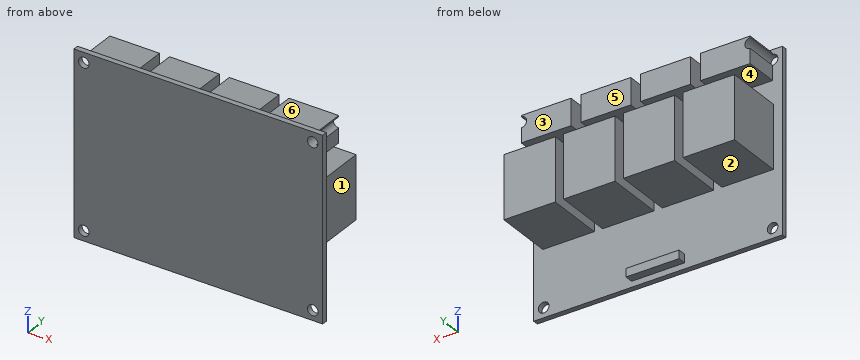
from build123d import *

# Parameters (mm, degrees)
SKETCH1_W              = 75
SKETCH1_H              = 55
PCB_DEPTH              = 1.6
RELAY_1_START          = 1.6
SKETCH2_W              = 15.5
SKETCH2_H              = 19
RELAY_1_DEPTH          = 17.4
TERMINAL_1_START       = 1.6
SKETCH3_W              = 15
SKETCH3_H              = 8
TERMINAL_1_DEPTH       = 10
RELAY_2_START          = 1.6
SKETCH4_W              = 15.5
SKETCH4_H              = 19
RELAY_2_DEPTH          = 17.4
TERMINAL_2_START       = 1.6
SKETCH5_W              = 15
SKETCH5_H              = 8
TERMINAL_2_DEPTH       = 10
RELAY_3_START          = 1.6
SKETCH6_W              = 15.5
SKETCH6_H              = 19
RELAY_3_DEPTH          = 17.4
TERMINAL_3_START       = 1.6
SKETCH7_W              = 15
SKETCH7_H              = 8
TERMINAL_3_DEPTH       = 10
RELAY_4_START          = 1.6
SKETCH8_W              = 15.5
SKETCH8_H              = 19
RELAY_4_DEPTH          = 17.4
TERMINAL_4_START       = 1.6
SKETCH9_W              = 15
SKETCH9_H              = 8
TERMINAL_4_DEPTH       = 10
HEADER_START           = 1.6
SKETCH10_W             = 16
SKETCH10_H             = 2.5
HEADER_DEPTH           = 2.5
MOUNT_HOLES_DEPTH      = 51.23445033
MOUNT_HOLES_DEPTH_BACK = 51.23445033
SKETCH11_R             = 1.6


with BuildPart() as part:
    # Sketch1 → PCB (new body)
    with BuildSketch(Plane(origin=(0, 0, 0), x_dir=(1, 0, 0), z_dir=(0, 1, 0))):
        Rectangle(SKETCH1_W, SKETCH1_H)
    extrude(amount=PCB_DEPTH)

    # Sketch2 → Relay_1 (add)
    with BuildSketch(Plane(origin=(0, 0, 0), x_dir=(1, 0, 0), z_dir=(0, 1, 0)).offset(RELAY_1_START)):
        with Locations((-27, -2)):
            Rectangle(SKETCH2_W, SKETCH2_H)
    extrude(amount=RELAY_1_DEPTH)

    # Sketch3 → Terminal_1 (add)
    with BuildSketch(Plane(origin=(0, 0, 0), x_dir=(1, 0, 0), z_dir=(0, 1, 0)).offset(TERMINAL_1_START)):
        with Locations((-27, -22.5)):
            Rectangle(SKETCH3_W, SKETCH3_H)
    extrude(amount=TERMINAL_1_DEPTH)

    # Sketch4 → Relay_2 (add)
    with BuildSketch(Plane(origin=(0, 0, 0), x_dir=(1, 0, 0), z_dir=(0, 1, 0)).offset(RELAY_2_START)):
        with Locations((-9, -2)):
            Rectangle(SKETCH4_W, SKETCH4_H)
    extrude(amount=RELAY_2_DEPTH)

    # Sketch5 → Terminal_2 (add)
    with BuildSketch(Plane(origin=(0, 0, 0), x_dir=(1, 0, 0), z_dir=(0, 1, 0)).offset(TERMINAL_2_START)):
        with Locations((-9, -22.5)):
            Rectangle(SKETCH5_W, SKETCH5_H)
    extrude(amount=TERMINAL_2_DEPTH)

    # Sketch6 → Relay_3 (add)
    with BuildSketch(Plane(origin=(0, 0, 0), x_dir=(1, 0, 0), z_dir=(0, 1, 0)).offset(RELAY_3_START)):
        with Locations((9, -2)):
            Rectangle(SKETCH6_W, SKETCH6_H)
    extrude(amount=RELAY_3_DEPTH)

    # Sketch7 → Terminal_3 (add)
    with BuildSketch(Plane(origin=(0, 0, 0), x_dir=(1, 0, 0), z_dir=(0, 1, 0)).offset(TERMINAL_3_START)):
        with Locations((9, -22.5)):
            Rectangle(SKETCH7_W, SKETCH7_H)
    extrude(amount=TERMINAL_3_DEPTH)

    # Sketch8 → Relay_4 (add)
    with BuildSketch(Plane(origin=(0, 0, 0), x_dir=(1, 0, 0), z_dir=(0, 1, 0)).offset(RELAY_4_START)):
        with Locations((27, -2)):
            Rectangle(SKETCH8_W, SKETCH8_H)
    extrude(amount=RELAY_4_DEPTH)

    # Sketch9 → Terminal_4 (add)
    with BuildSketch(Plane(origin=(0, 0, 0), x_dir=(1, 0, 0), z_dir=(0, 1, 0)).offset(TERMINAL_4_START)):
        with Locations((27, -22.5)):
            Rectangle(SKETCH9_W, SKETCH9_H)
    extrude(amount=TERMINAL_4_DEPTH)

    # Sketch10 → Header (add)
    with BuildSketch(Plane(origin=(0, 0, 0), x_dir=(1, 0, 0), z_dir=(0, 1, 0)).offset(HEADER_START)):
        with Locations((0, 24.5)):
            Rectangle(SKETCH10_W, SKETCH10_H)
    extrude(amount=HEADER_DEPTH)

    # Sketch11 → Mount_Holes (cut, two sides: drawn at the far end of the back side and taken through both)
    with BuildSketch(Plane(origin=(0, 0, 0), x_dir=(1, 0, 0), z_dir=(0, 1, 0)).offset(-MOUNT_HOLES_DEPTH_BACK)):
        with Locations(Location((-34.5, 24.5, 0), (0, 0, 90))):
            Circle(SKETCH11_R)
        with Locations(Location((-34.5, -24.5, 0), (0, 0, 270))):
            Circle(SKETCH11_R)
        with Locations(Location((34.5, 24.5, 0), (0, 0, 90))):
            Circle(SKETCH11_R)
        with Locations(Location((34.5, -24.5, 0), (0, 0, 270))):
            Circle(SKETCH11_R)
    extrude(amount=MOUNT_HOLES_DEPTH + MOUNT_HOLES_DEPTH_BACK, mode=Mode.SUBTRACT)


solid = part.part
Geometry: final body of the model. Coordinates: model frame, mm. Face numbers are marked on the shaded views. A direction names the side the tool comes from. Coordinates: 2 decimals unless noted, no trailing zeros. Order: outer loops, then holes, each group sorted by start corner. A loop starts at its lowest first (then second) coordinate and runs counter-clockwise, first axis right, second up.
(1) Access query for the marked faces 1, 2 and 3. Directions: +Z, -Z, +X, -X, +Y, -Y. A direction counts if a zero-diameter tool reaches every point of the face in a straight line with its end or side. Return the directions, or none.
(2) Material intervals for probe 1 along X at (y, z) = (3.5, 24.5); probe 2 along X at (y, z) = (2.5, 0.5); probe 3 along X at (y, z) = (1.25, -24.5), sorted ascending.
(3) Draft query along Z for the marked faces 4, 5 and 6. Return one class per face: pulls with the +Z half, pulls with the -Z half, needs draft (parallel to the pull), parting line crosses it, or undercut.
(4) First-contact query: pin 1 (1 mm diameter, centred on x = 0.5, y = 11.5, fed in from -Z); pin 2 (5 mm diameter, centred on x = -12.5, y = 8, fed in from -Z); pin 3 (2.5 mm diameter, centred on y = 5.5, z = 23.5, fed in from -X); pin 4 (1.5 mm diameter, centred on x = 8.5, z = -18.5, fed in from +Y). Flat tips, straight axial feed; report the tip coordinate or a pass-through.
(5) Section query C-C (x = 21). Return the cut outline in (y, z), plus the area to 3 significant figures.
(6) Section query B-B (z = 24.5). Return the cut outline in (x, y).
(7) Section query A-A (y = 13.5). Return the cut outline in (x, z), plus the area to 3 significant figures.
(8) Section query D-D (z = -5). Return the cut outline in (x, y), plus the area to 3 significant figures.
Solution:
1. face 1: +Z, -Z, +X, +Y
1. face 2: -Z, +X, -X, +Y
1. face 3: +Z, +X, -X, +Y
2. probe 1: x = -32.9 to -19.5, -16.5 to -1.5, 1.5 to 16.5, 19.5 to 32.9
2. probe 2: x = -34.75 to -19.25, -16.75 to -1.25, 1.25 to 16.75, 19.25 to 34.75
2. probe 3: x = -37.5 to -36.1, -32.9 to 32.9, 36.1 to 37.5
3. face 4: undercut
3. face 5: needs draft
3. face 6: pulls with the +Z half
4. pin 1: passes through
4. pin 2: stops at z = -7.5
4. pin 3: stops at x = -34.5
4. pin 4: stops at y = 1.6
5. outline: (0, -27.5) - (1.6, -27.5) - (1.6, -7.5) - (19, -7.5) - (19, 11.5) - (1.6, 11.5) - (1.6, 18.5) - (11.6, 18.5) - (11.6, 26.5) - (1.6, 26.5) - (1.6, 27.5) - (0, 27.5) - close
5. area: 499 mm2
6. outline: (-37.5, 0) - (-36.1, 0) - (-36.1, 1.6) - (-37.5, 1.6) - close; (-32.9, 0) - (32.9, 0) - (32.9, 11.6) - (19.5, 11.6) - (19.5, 1.6) - (16.5, 1.6) - (16.5, 11.6) - (1.5, 11.6) - (1.5, 1.6) - (-1.5, 1.6) - (-1.5, 11.6) - (-16.5, 11.6) - (-16.5, 1.6) - (-19.5, 1.6) - (-19.5, 11.6) - (-32.9, 11.6) - close; (36.1, 0) - (37.5, 0) - (37.5, 1.6) - (36.1, 1.6) - close
7. outline: (-34.75, -7.5) - (-19.25, -7.5) - (-19.25, 11.5) - (-34.75, 11.5) - close; (-16.75, -7.5) - (-1.25, -7.5) - (-1.25, 11.5) - (-16.75, 11.5) - close; (1.25, -7.5) - (16.75, -7.5) - (16.75, 11.5) - (1.25, 11.5) - close; (19.25, -7.5) - (34.75, -7.5) - (34.75, 11.5) - (19.25, 11.5) - close
7. area: 1,180 mm2
8. outline: (-37.5, 0) - (37.5, 0) - (37.5, 1.6) - (34.75, 1.6) - (34.75, 19) - (19.25, 19) - (19.25, 1.6) - (16.75, 1.6) - (16.75, 19) - (1.25, 19) - (1.25, 1.6) - (-1.25, 1.6) - (-1.25, 19) - (-16.75, 19) - (-16.75, 1.6) - (-19.25, 1.6) - (-19.25, 19) - (-34.75, 19) - (-34.75, 1.6) - (-37.5, 1.6) - close
8. area: 1,200 mm2
